The listing builds one solid part. Answer for the finished solid, in the listing's coordinates (mm). A direction names the side the tool comes from. Give positions to 0.01 mm unless a question says otherwise; leave off trailing zeros. Order: outer loops, then holes, each group sorted by start corner. A loop starts at its lowest first (then second) coordinate and runs counter-clockwise, first axis right, second up. Notation, with made-up numbers: (60.25, 23.5) - (78.25, 23.5) arc R14 cw to (78.25, 48.5) - close; hole circle Ø10 at (82, -4.75). An arc over 180 degrees is marked (long way). Answer as CSV lines item,"result". Start each with the question number.
1. Section C-C on x = -98.5 is taken. Give the vertices of the cut face in (y, z), and give its area (3 significant figures).
2. Which of the six approach directions +Z, -Z, +X, -X, +Y, -Y give full straight-line access (tool end or side, diameter ignored) to faces 1 (the flat face through (-120.209, -134.522, 12704.45)), 2 (the flat face through (-35.13, 0.8, 12704.49)), 3 (the flat face through (-105.88, -118.51, 12704.49))?
3. Determine the mould class of faces 4 (the cylindrical face through (-70.398, 29.084, 12704.485)), 5 (the flat face through (-0.57, 44.39, 12826.5)), 6 (the flat face through (-103.723, 45.792, 12578.968)) for opening direction X: +X half, -X half, draft (parallel to the pull), parting line (faces both ways), or undercut.
4. Consider line 1 along Y through (x, z) = (-113, 12743); line 2 along Y through (x, z) = (-115.5, 12592.5); line 3 along X through (y, z) = (-114, 12632). Determine where each line is inside the solid, lowest interval first. Write a range as [from, to].
5. Section A-A on z = 12704 is taken. Give the vertices of the cut face in (x, y).
6. Section D-D on y = -30 is taken. Give the vertices of the cut face in (x, z), and give its area (3 significant figures).
7. Section B-B on y = 65 is taken. Give the vertices of the cut face in (x, z), and give its area (3 significant figures).
8. Flat-ended cylindrical pins translate along their axes: pin 1 (1 mm diameter, centred on x = -127.5, z = 12717.5, fed in from -Y); pin 2 (1.5 mm diameter, centred on x = -64.5, z = 12687.5, fed in from -Y); pin 3 (8 mm diameter, centred on y = -76, z = 12773, fed in from -X). Find the tip coordinate at first contact, or state that the pin passes through.
from build123d import *

# Parameters (mm, degrees)
EXTRUDE_2_DEPTH = 250
CHAMFER_1_SIZE  = 2.5


with BuildPart() as part:
    # 草圖1 → 填料-伸長2 (new body)
    with BuildSketch(Plane(origin=(1e-09, -1e-09, 12827.735128457), x_dir=(1, 0, 0), z_dir=(0, 0, 1))):
        with BuildLine():
            Line((-112.117770632, -75.640230505), (-108.139732902, -53.167558993))
            ThreePointArc((-108.139732902, -53.167558993), (-128.285417164, -21.997695969), (-91.181469021, -22.837926636))
            Line((-91.181469021, -22.837926636), (-74.915186503, -8.426224475))
            ThreePointArc((-74.915186503, -8.426224475), (-69.768626313, 29.297285814), (-43.57987489, 1.662170304))
            Line((-43.57987489, 1.662170304), (-26.446012397, -0.086903016))
            ThreePointArc((-26.446012397, -0.086903016), (-11.209248537, 23.49241234), (13.857582965, 10.851326786))
            Line((13.857582965, 10.851326786), (-13.929514572, 82.148324057))
            Line((-13.929514572, 82.148324057), (-196.933065463, 10.825018546))
            Line((-196.933065463, 10.825018546), (-137.638404215, -141.315063571))
            Line((-137.638404215, -141.315063571), (-102.351415407, -127.562408658))
            Line((-102.351415407, -127.562408658), (-108.57535624, -111.5928281))
            ThreePointArc((-108.57535624, -111.5928281), (-141.904281803, -96.725915639), (-112.117770632, -75.640230505))
        make_face()
    extrude(amount=-EXTRUDE_2_DEPTH)

    # 導角1
    chamfer_1_edges = [part.edges().sort_by_distance(p)[0] for p in [
        (-119.99490981, -134.438736116, 12827.735128457),
        (-167.285734839, -65.245022514, 12827.735128457),
        (-105.431290017, 46.4866713, 12827.735128457),
        (-0.035965803, 46.49982542, 12827.735128457),
        (-0.035965803, 46.49982542, 12577.735128457),
        (-102.351415406, -127.562408659, 12702.735128457),
        (-137.638404215, -141.315063573, 12702.735128457),
        (-196.933065463, 10.825018545, 12702.735128457),
        (-13.929514572, 82.148324055, 12702.735128457),
        (-105.431290017, 46.4866713, 12577.735128457),
        (-167.285734839, -65.245022514, 12577.735128457),
        (-119.99490981, -134.438736116, 12577.735128457),
    ]]
    chamfer(chamfer_1_edges, length=CHAMFER_1_SIZE)


solid = part.part
Checks:
1,outline,"(-14.65, 12577.74) - (46.5, 12577.74) - (49.19, 12580.24) - (49.19, 12825.24) - (46.5, 12827.74) - (-14.65, 12827.74) - close"
1,area,"16,000 mm²"
2,face 1,"+Z, -Z, +X, -Y"
2,face 2,"+Z, -Z, -Y"
2,face 3,"+Z, -Z, +X"
3,face 4,"undercut"
3,face 5,"+X half"
3,face 6,"-X half"
4,line 1,"y = [-131.71, -114.08], [-75.25, -53.02], [-11.47, 43.54]"
4,line 2,"y = [-132.69, -114.93], [-74.4, -52.5], [-11.99, 42.56]"
4,line 3,"x = [-148.28, -129.2], [-112.81, -107.64]"
5,outline,"(-196.03, 8.5) - (-138.55, -138.99) - (-135.31, -140.41) - (-104.68, -128.47) - (-103.26, -125.23) - (-108.58, -111.59) arc R21 cw (long way) to (-112.12, -75.64) - (-108.14, -53.17) arc R21 cw (long way) to (-91.18, -22.84) - (-74.92, -8.43) arc R21.11 cw (long way) to (-43.58, 1.66) - (-26.45, -0.09) arc R21 cw to (13.86, 10.85) - (-13.02, 79.82) - (-16.26, 81.24) - (-194.6, 11.73) - close"
6,outline,"(-181.02, 12580.24) - (-178.34, 12577.74) - (-130.84, 12577.74) - (-130.84, 12827.74) - (-178.34, 12827.74) - (-181.02, 12825.24) - close"
6,area,"12,500 mm²"
7,outline,"(-57.93, 12580.24) - (-51.04, 12577.74) - (-9.93, 12577.74) - (-7.25, 12580.24) - (-7.25, 12825.24) - (-9.93, 12827.74) - (-51.04, 12827.74) - (-57.93, 12825.24) - close"
7,area,"12,600 mm²"
8,pin 1,"stops at y = -137.56"
8,pin 2,"stops at y = 30.22"
8,pin 3,"stops at x = -164.65"
